```python
from build123d import *

# Parameters (mm, degrees)
SKETCH1_R             = 1.6
SKETCH1_R_2           = 1.25
BOSS_EXTRUDE1_DEPTH   = 2.25
BOSS_EXTRUDE1_2_DEPTH = 2.25
BOSS_EXTRUDE1_3_DEPTH = 2.25
BOSS_EXTRUDE1_4_DEPTH = 2.25
SKETCH2_R             = 1.25
BOSS_EXTRUDE2_DEPTH   = 1.5
FILLET1_R             = 1


with BuildPart() as part:
    # Sketch1 → Boss-Extrude1 (new body)
    with BuildSketch(Plane.XY):
        with Locations((-12.15, 12.15)):
            Circle(SKETCH1_R)
        with Locations((-12.15, 12.15)):
            Circle(SKETCH1_R_2, mode=Mode.SUBTRACT)
    extrude(amount=BOSS_EXTRUDE1_DEPTH)



with BuildPart() as body_2:
    # Sketch1 → Boss-Extrude1 2 (new body)
    with BuildSketch(Plane.XY):
        with Locations((12.15, 12.15)):
            Circle(SKETCH1_R)
        with Locations((12.15, 12.15)):
            Circle(SKETCH1_R_2, mode=Mode.SUBTRACT)
    extrude(amount=BOSS_EXTRUDE1_2_DEPTH)


with BuildPart() as body_3:
    # Sketch1 → Boss-Extrude1 3 (new body)
    with BuildSketch(Plane.XY):
        with Locations((12.15, -12.15)):
            Circle(SKETCH1_R)
        with Locations((12.15, -12.15)):
            Circle(SKETCH1_R_2, mode=Mode.SUBTRACT)
    extrude(amount=BOSS_EXTRUDE1_3_DEPTH)


with BuildPart() as body_4:
    # Sketch1 → Boss-Extrude1 4 (new body)
    with BuildSketch(Plane.XY):
        with Locations((-12.15, -12.15)):
            Circle(SKETCH1_R)
        with Locations((-12.15, -12.15)):
            Circle(SKETCH1_R_2, mode=Mode.SUBTRACT)
    extrude(amount=BOSS_EXTRUDE1_4_DEPTH)


with BuildPart() as part_1:
    add(part.part)

    add(body_2.part)  # Boss-Extrude2 merges body 2

    add(body_3.part)  # Boss-Extrude2 merges body 3

    add(body_4.part)  # Boss-Extrude2 merges body 4
    # Sketch2 → Boss-Extrude2 (add)
    with BuildSketch(Plane.XY.offset(2.25)):
        with BuildLine():
            Line((12.15, 13.75), (-12.15, 13.75))
            ThreePointArc((-12.15, 13.75), (-13.28137085, 13.28137085), (-13.75, 12.15))
            Line((-13.75, 12.15), (-13.75, -12.15))
            ThreePointArc((-13.75, -12.15), (-13.28137085, -13.28137085), (-12.15, -13.75))
            Line((-12.15, -13.75), (-0.025, -13.75))
            Line((-0.025, -13.75), (-0.025, -10.1))
            Line((-0.025, -10.1), (10.975, -10.1))
            Line((10.975, -10.1), (10.975, -11.064009669))
            ThreePointArc((10.975, -11.064009669), (11.566904811, -13.639966443), (13.75, -12.15))
            Line((13.75, -12.15), (13.75, 12.15))
            ThreePointArc((13.75, 12.15), (13.28137085, 13.28137085), (12.15, 13.75))
        make_face()
        with Locations((-12.15, 12.15)):
            Circle(SKETCH2_R, mode=Mode.SUBTRACT)
        with Locations((12.15, 12.15)):
            Circle(SKETCH2_R, mode=Mode.SUBTRACT)
        with Locations((-12.15, -12.15)):
            Circle(SKETCH2_R, mode=Mode.SUBTRACT)
        with Locations((12.15, -12.15)):
            Circle(SKETCH2_R, mode=Mode.SUBTRACT)
    extrude(amount=BOSS_EXTRUDE2_DEPTH)

    # Fillet1
    # the kernel refuses this fillet: 1 mm, written as the material it adds along each edge
    with BuildSketch(Plane(origin=(10.975, -10.1, 2.25), x_dir=(-1, 0, 0), z_dir=(0, 0, 1)), Plane(origin=(-0.025, -10.1, 2.25), x_dir=(0, -1, 0), z_dir=(0, 0, 1))) as fillet1_piece_1:
        with BuildLine():
            CenterArc((FILLET1_R, FILLET1_R), FILLET1_R, 180, 90)
            Line((0, FILLET1_R), (0, 0))
            Line((0, 0), (FILLET1_R, 0))
        make_face()
    extrude(amount=1.5)


solid = part_1.part
```
Verification items for the finished model (mm, model axes). A direction names the side the tool comes from. Give positions to 0.01 mm unless a question says otherwise; leave off trailing zeros. Order: outer loops, then holes, each group sorted by start corner. A loop starts at its lowest first (then second) coordinate and runs counter-clockwise, first axis right, second up. Notation, with made-up numbers: M 71.5,18 L 80.5,18 A9 cw 80.5,27 Z; hole C 66.25,-2.75 d8. An arc over 180 degrees is marked long. Answer in a Markdown table with one row per item. Add a question column.
Item 1: Section check A-A, the plane z = 0.35. Enter the section's corners in (x, y), and give its area (3 significant figures).
Item 2: Scan lines: probe 1 along Y at (x, z) = (-12.15, 2.4); probe 2 along Y at (x, z) = (-12.15, 0.8); probe 3 along Y at (x, z) = (-11.5, 0.6). Record each from-to range of solid material in increasing order. Write a range as from..to.
Item 3: Section check B-B, the plane z = 3. Enter the section's corners in (x, y) (3 decimals), and give its area (3 significant figures).
Item 4: Mould release check, pull along X, two halves, no side actions. Record for faces 4 (the flat face through (13, 11, 0)), 5 (the flat face through (-13.75, 0, 3)), 6 (the cylindrical face through (10.68, -10.39, 2.99)): released by +X, released by -X, zero draft, split by the parting line, or undercut.
Item 5: Section check C-C, the plane x = 11.5. Enter the section's corners in (y, z).
Item 6: Section check D-D, the plane y = 8. Enter the section's corners in (x, z).
Item 7: Tool access check on faces 1 (the cylindrical face through (11.88, -13.37, 1.85)), 2 (the flat face through (0, 0, 2.25)), 3 (the flat face through (-0.025, -12, 3)). Record the directions out of +Z, -Z, +X, -X, +Y, -Y that give a thin tool (end or side, any length) a straight path to the whole face; none if there is none.
Item 8: Gauge pin test, flat ends, axial feed: pin 1 (0.8 mm diameter, centred on x = 4.5, z = 3, fed in from -Y); pin 2 (3 mm diameter, centred on x = 12.15, y = 12.15, fed in from +Z); pin 3 (8 mm diameter, centred on x = 6.5, y = 6.5, fed in from -Z); pin 4 (1 mm diameter, centred on x = -10.5, z = 1, fed in from -Y). Record the tip position at first contact, or that the pin passes through.
Filled sheet:
| question | item | result |
|---|---|---|
| 1 | outline | C -12.15,-12.15 d3.2; C -12.15,12.15 d3.2; C 12.15,-12.15 d3.2; C 12.15,12.15 d3.2; hole C -12.15,-12.15 d2.5; hole C -12.15,12.15 d2.5; hole C 12.15,-12.15 d2.5; hole C 12.15,12.15 d2.5 |
| 1 | area | 12.5 mm^2 |
| 2 | probe 1 | y = -13.75..-13.4, -10.9..10.9, 13.4..13.75 |
| 2 | probe 2 | y = -13.75..-13.4, -10.9..-10.55, 10.55..10.9, 13.4..13.75 |
| 2 | probe 3 | y = -13.61..-13.22, -11.08..-10.69, 10.69..11.08, 13.22..13.61 |
| 3 | outline | M -13.75,-12.15 A1.6 ccw -12.15,-13.75 L -0.025,-13.75 L -0.025,-11.1 A1 cw 0.975,-10.1 L 9.975,-10.1 A1 cw 10.974,-11.065 A1.6 ccw long 13.75,-12.15 L 13.75,12.15 A1.6 ccw 12.15,13.75 L -12.15,13.75 A1.6 ccw -13.75,12.15 Z; hole C -12.15,-12.15 d2.5; hole C -12.15,12.15 d2.5; hole C 12.15,-12.15 d2.5; hole C 12.15,12.15 d2.5 |
| 3 | area | 695 mm^2 |
| 4 | face 4 | zero draft |
| 4 | face 5 | released by -X |
| 4 | face 6 | undercut |
| 5 | outline | M -13.61,0 L -13.22,0 L -13.22,3.75 L -13.61,3.75 Z; M -11.08,0 L -10.69,0 L -10.69,2.25 L 10.69,2.25 L 10.69,0 L 11.08,0 L 11.08,3.75 L -11.08,3.75 Z; M 13.22,0 L 13.61,0 L 13.61,2.25 L 13.75,2.25 L 13.75,3.75 L 13.22,3.75 Z |
| 6 | outline | M -13.75,2.25 L 13.75,2.25 L 13.75,3.75 L -13.75,3.75 Z |
| 7 | face 1 | +Z, -Z |
| 7 | face 2 | -Z |
| 7 | face 3 | +Z, -Z, -Y |
| 8 | pin 1 | stops at y = -10.1 |
| 8 | pin 2 | stops at z = 3.75 |
| 8 | pin 3 | stops at z = 2.25 |
| 8 | pin 4 | stops at y = -13.26 |
